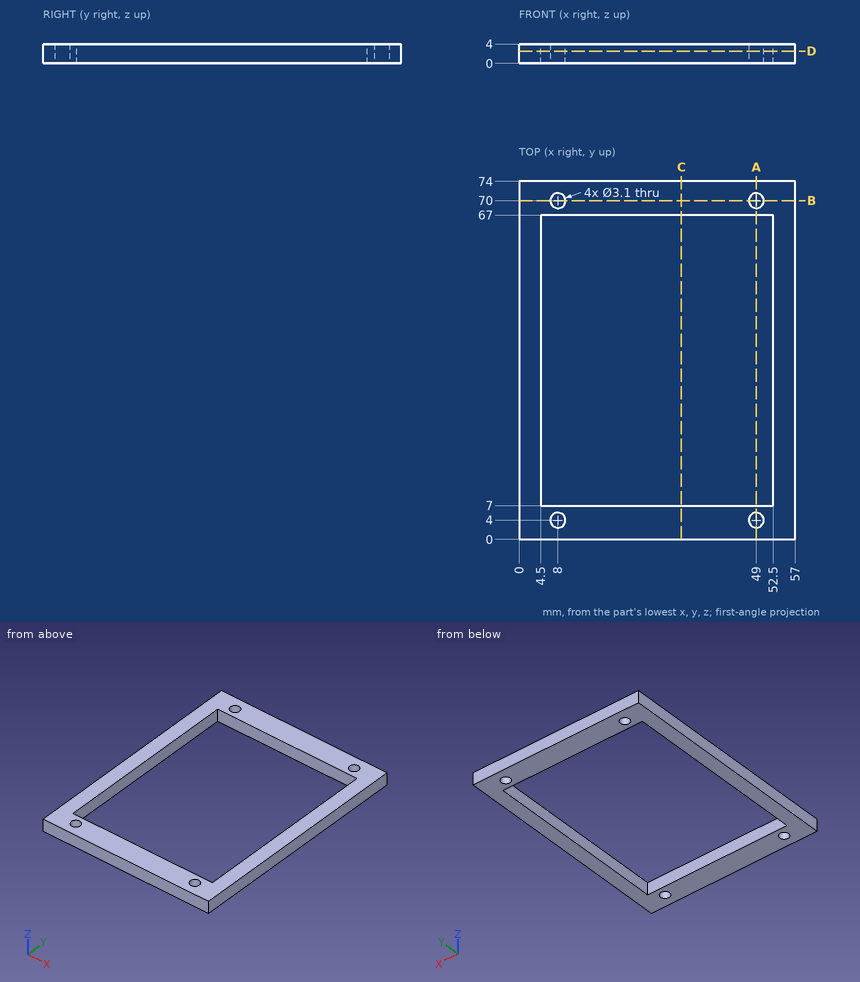
Input: dimensioned drawing with shaded views. Units: mm. Origin: part minimum x, y, z. Coordinates: 2 decimals unless noted, no trailing zeros. Order: outer loops, then holes, each group sorted by start corner. A loop starts at its lowest first (then second) coordinate and runs counter-clockwise, first axis right, second up.
Item 1: Section query B-B (y = 70). Output: boundary loops of the cut face in (x, z), then the cut area to 3 significant figures.
Answer:
outline: (0, 0) - (6.45, 0) - (6.45, 4) - (0, 4) - close; (9.55, 0) - (47.45, 0) - (47.45, 4) - (9.55, 4) - close; (50.55, 0) - (57, 0) - (57, 4) - (50.55, 4) - close
area: 203 mm2
Item 2: Material intervals for line 1 along Y through (x, z) = (49, 2.05); line 2 along X through (y, z) = (70, 1.35); line 3 along Y through (x, z) = (28, 1.5), sorted ascending.
Answer:
line 1: y = 0 to 2.45, 5.55 to 7, 67 to 68.45, 71.55 to 74
line 2: x = 0 to 6.45, 9.55 to 47.45, 50.55 to 57
line 3: y = 0 to 7, 67 to 74
Item 3: Section query D-D (z = 2.55). Output: boundary loops of the cut face in (x, y), then the cut area to 3 significant figures.
Answer:
outline: (0, 0) - (57, 0) - (57, 74) - (0, 74) - close; hole (4.5, 7) - (52.5, 7) - (52.5, 67) - (4.5, 67) - close; hole circle Ø3.1 at (8, 4); hole circle Ø3.1 at (8, 70); hole circle Ø3.1 at (49, 4); hole circle Ø3.1 at (49, 70)
area: 1,310 mm2
Item 4: Section query A-A (x = 49). Output: boundary loops of the cut face in (y, z), then the cut area to 3 significant figures.
Answer:
outline: (0, 0) - (2.45, 0) - (2.45, 4) - (0, 4) - close; (5.55, 0) - (7, 0) - (7, 4) - (5.55, 4) - close; (67, 0) - (68.45, 0) - (68.45, 4) - (67, 4) - close; (71.55, 0) - (74, 0) - (74, 4) - (71.55, 4) - close
area: 31.2 mm2
Item 5: Section query C-C (x = 33.5). Output: boundary loops of the cut face in (y, z), then the cut area to 3 significant figures.
Answer:
outline: (0, 0) - (7, 0) - (7, 4) - (0, 4) - close; (67, 0) - (74, 0) - (74, 4) - (67, 4) - close
area: 56.0 mm2
Item 6: Contact query for flat-ended pins moving along their axis: P1, Ø3, axis at x = 8, y = 4, coming from the +Z side (1 decimal); P2, Ø3.5, axis at x = 49, y = 4, coming from the +Z side. Output: stop coordinate, or through.
Answer:
P1: passes through
P2: stops at z = 4
